Work out the finished part from the listing and answer in its coordinate system (mm). A direction names the side the tool comes from. Give positions to 0.01 mm unless a question says otherwise; leave off trailing zeros. Order: outer loops, then holes, each group sorted by start corner. A loop starts at its lowest first (then second) coordinate and runs counter-clockwise, first axis right, second up. Notation, with made-up numbers: (16, -16) - (41, -16) arc R11 ccw to (41, 1) - close; hole circle Ø5 at (3, -37.75). An arc over 180 degrees is marked (long way). Write each question's results on one line, items separated by ' | '.
from build123d import *

# Parameters (mm, degrees)
F1_DEPTH = 34.925
F2_R     = 2.54
F3_DEPTH = 25.4
F4_R     = 5.08
F5_R     = 3.175
F6_W     = 50.8
F6_H     = 25.4
F7_DEPTH = 6.4008


with BuildPart() as f1:
    # F0 (on Front) → F1 (new body)
    with BuildSketch(Plane.XZ):
        Polygon((-12.7, 0), (0, 0), (12.7, 0), (44.45, 0), (44.45, 3.175), (31.75, 3.175), (31.75, 9.525), (-31.75, 9.525), (-31.75, 3.175), (-44.45, 3.175), (-44.45, 0), align=None)
    extrude(amount=F1_DEPTH)

    # F2 (on face) → F3 (cut)
    with BuildSketch(Plane(origin=(0, 0, 0), x_dir=(1, 0, 0), z_dir=(0, 0, -1))):
        with Locations((-38.1, 25.4)):
            Circle(F2_R)
        with Locations((-38.1, 9.525)):
            Circle(F2_R)
        with Locations((38.1, 25.4)):
            Circle(F2_R)
        with Locations((38.1, 9.525)):
            Circle(F2_R)
    extrude(amount=-F3_DEPTH, mode=Mode.SUBTRACT)

    # F4
    f4_edges = [f1.edges().sort_by_distance(p)[0] for p in [
        (-44.45, -34.925, 1.5875),
        (44.45, -34.925, 1.5875),
        (44.45, 0, 1.5875),
        (-44.45, 0, 1.5875),
        (31.75, 0, 6.35),
        (-31.75, 0, 6.35),
        (31.75, -34.925, 6.35),
        (-31.75, -34.925, 6.35),
    ]]
    fillet(f4_edges, radius=F4_R)

    # F5
    f5_edges = [f1.edges().sort_by_distance(p)[0] for p in [
        (-30.262102, -33.437102, 9.525),
    ]]
    fillet(f5_edges, radius=F5_R)

    # F6 (on face) → F7 (cut)
    with BuildSketch(Plane(origin=(0, 0, 0), x_dir=(1, 0, 0), z_dir=(0, 0, -1))):
        with Locations((0, 17.4625)):
            Rectangle(F6_W, F6_H)
    extrude(amount=-F7_DEPTH, mode=Mode.SUBTRACT)


solid = f1.part
1. A tool of negligible diameter and unlimited length cuts with its end or side. For faces 1 (the face through (31.75, -17, 5)), 2 (the face through (-30.2, -33.5, 4.7)), 3 (the face through (-31.75, -17, 5)), 4 (the face through (25.4, -17, 3)), from which of +Z, -Z, +X, -X, +Y, -Y can it reach the whole face along a straight path? Write none if from no direction.
Answer list:
face 1: +Z, +X, +Y, -Y | face 2: +Z, -X, -Y | face 3: +Z, -X, +Y, -Y | face 4: -Z
2. Straight lines are drawn through the part: line 1 (Y direction, x = 38.1, z = 1.4) (3 decimals); line 2 (X direction, y = -25.4, z = 1.9); line 3 (Y direction, x = 7, z = 5.5) (1 decimal). For each, find the intervals that lie inside material, in ascending order. Write a range as [from, to].
Answer list:
line 1: [-34.925, -27.94], [-22.86, -12.065], [-6.985, 0] | line 2: [-44.45, -40.64], [-35.56, -25.4], [25.4, 35.56], [40.64, 44.45] | line 3: [-34.9, -30.2], [-4.8, 0]
3. A cutting plane is placed at A-A, the plane x = 38.1. Write down the section's boundary in (y, z) (3 decimals).
Answer list:
outline: (-34.925, 0) - (-27.94, 0) - (-27.94, 3.175) - (-34.925, 3.175) - close; (-22.86, 0) - (-12.065, 0) - (-12.065, 3.175) - (-22.86, 3.175) - close; (-6.985, 0) - (0, 0) - (0, 3.175) - (-6.985, 3.175) - close
4. A cutting plane is placed at D-D, the plane y = -14.5. Write down the section's boundary in (x, z) (3 decimals).
Answer list:
outline: (-44.45, 0) - (-25.4, 0) - (-25.4, 6.401) - (25.4, 6.401) - (25.4, 0) - (44.45, 0) - (44.45, 3.175) - (31.75, 3.175) - (31.75, 6.35) arc R3.175 ccw to (28.575, 9.525) - (-28.575, 9.525) arc R3.175 ccw to (-31.75, 6.35) - (-31.75, 3.175) - (-44.45, 3.175) - close
5. Given P1, Ø3, axis at x = -38.1, y = -9.525, coming from the +Z side; P2, Ø1.6, axis at y = -21.5, z = 5, coming from the +X side; P3, Ø6, axis at x = 38.1, y = -25.4, coming from the +Z side (3 decimals); P4, Ø2.5, axis at y = -22.5, z = 5, coming from the -X side, each flat-ended and moving along its own axis, determine where each tip first touches the part or whether it passes through.
Answer list:
P1: through | P2: x = 31.75 | P3: z = 3.175 | P4: x = -31.75
6. A cutting plane is placed at B-B, the plane y = -25.4. Write down the section's boundary in (x, z) (3 decimals), then the cut area to 3 significant figures.
Answer list:
outline: (-44.45, 0) - (-40.64, 0) - (-40.64, 3.175) - (-44.45, 3.175) - close; (-35.56, 0) - (-25.4, 0) - (-25.4, 6.401) - (25.4, 6.401) - (25.4, 0) - (35.56, 0) - (35.56, 3.175) - (31.75, 3.175) - (31.75, 6.35) arc R3.175 ccw to (28.575, 9.525) - (-28.575, 9.525) arc R3.175 ccw to (-31.75, 6.35) - (-31.75, 3.175) - (-35.56, 3.175) - close; (40.64, 0) - (44.45, 0) - (44.45, 3.175) - (40.64, 3.175) - close | area: 324 mm^2
7. Determine the mould class of faces 5 (the face through (35.562, -9.637, 1.565)), 6 (the face through (-1, -34.925, 3)), 7 (the face through (43.001, -1.528, 1.61)) for opening direction Y: +Y half, -Y half, draft (parallel to the pull), parting line (faces both ways), or undercut.
Answer list:
face 5: undercut | face 6: -Y half | face 7: +Y half
